```python
from build123d import *

# Parameters (mm, degrees)
SKETCH1_R           = 12.5
SKETCH1_R_2         = 2.5
BOSS_EXTRUDE1_DEPTH = 127
CHAMFER1_SIZE       = 2


with BuildPart() as part:
    # Sketch1 → Boss-Extrude1 (new, symmetric)
    with BuildSketch(Plane.XY):
        Circle(SKETCH1_R)
        Circle(SKETCH1_R_2, mode=Mode.SUBTRACT)
    extrude(amount=BOSS_EXTRUDE1_DEPTH, both=True)

    # Chamfer1
    chamfer1_edges = [part.edges().sort_by_distance(p)[0] for p in [
        (-12.5, 0, -127),
        (-12.5, 0, 127),
        (-2.5, 0, -127),
        (-2.5, 0, 127),
    ]]
    chamfer(chamfer1_edges, length=CHAMFER1_SIZE)


solid = part.part
```
Here's how the part is built. I have some questions about the finished solid (model axes, mm). Coordinates: 2 decimals unless noted, no trailing zeros. Loops run counter-clockwise (first coordinate to the right, second up) from the corner with the lowest first, then second, coordinate; pieces in that order, holes last. Notation, with made-up numbers: (-22.75, 74) - (7.25, 74) arc R3 cw to (7.25, 79) - close; hole circle Ø3 at (10, -15.75). An arc over 180 degrees is marked (long way). Answer as CSV lines item,"result".
Q1. For pin 1 (1 mm diameter, centred on y = -8.5, z = -53.5, fed in from -X); pin 2 (6 mm diameter, centred on x = 0, y = 0, fed in from +Z); pin 3 (1 mm diameter, centred on y = -4, z = 25.5, fed in from +X), each with a flat end and sliding along its axis, tell me the tip position at first contact or that it passes through.
Response:
pin 1,"x = -9.6"
pin 2,"z = 125.5"
pin 3,"x = 12"
Q2. If I drill on L1, parallel to Y at x = 0, z = 9; L2, parallel to Y at x = 1.5, z = -8; L3, parallel to Z at x = -3.25, y = 0.75, over which ranges is the centre line in solid material (lowest first)? Write a range as [from, to].
Response:
L1,"[-12.5, -2.5], [2.5, 12.5]"
L2,"[-12.41, -2], [2, 12.41]"
L3,"[-125.84, 125.84]"
Q3. We'd pull the mould along Y, two halves only. Please class faces 1 (the face through (-2.083, -1.597, -125.125)), 2 (the face through (-0.54, -2.44, -1.75)), 3 (the face through (11.923, 3.755, 1.75)), 4 (the face through (5, 0, 127)): pulls with the +Y half, pulls with the -Y half, needs draft (parallel to the pull), parting line crosses it, or undercut.
Response:
face 1,"undercut"
face 2,"undercut"
face 3,"parting line crosses it"
face 4,"needs draft"
Q4. If we section it at A-A, the plane x = 0: Write out the boundary of the cut face in (y, z).
Response:
outline,"(-12.5, -125) - (-10.5, -127) - (-4.5, -127) - (-2.5, -125) - (-2.5, 125) - (-4.5, 127) - (-10.5, 127) - (-12.5, 125) - close; (2.5, -125) - (4.5, -127) - (10.5, -127) - (12.5, -125) - (12.5, 125) - (10.5, 127) - (4.5, 127) - (2.5, 125) - close"
Q5. If we section it at C-C, the plane z = -11.5: Write out the boundary of the cut face in (x, y), and give its area (3 significant figures).
Response:
outline,"circle Ø25 at (0, 0); hole circle Ø5 at (0, 0)"
area,"471 mm2"
